```python
from build123d import *

# Parameters (mm, degrees)
BOSS_EXTRUDE1_DEPTH                             = 4.7625
CUT_EXTRUDE1_DEPTH                              = 98.916706472
FILLET1_R                                       = 3
M2_5X0_45_TAPPED_HOLE1_D                        = 2.05
M4X0_7_TAPPED_HOLE1_D                           = 3.3
M4X0_7_TAPPED_HOLE1_DEPTH                       = 11.5
M4X0_7_TAPPED_HOLE1_TIP                         = 0.991420021
CSK_FOR_M3_FLAT_HEAD_MACHINE_SCREW1_D           = 3.4
CSK_FOR_M3_FLAT_HEAD_MACHINE_SCREW1_CSINK_D     = 6.3
CSK_FOR_M3_FLAT_HEAD_MACHINE_SCREW1_CSINK_ANGLE = 90
CUT_EXTRUDE2_DEPTH                              = 84.778552935
FILLET2_R                                       = 2


with BuildPart() as part:
    # Sketch1 → Boss-Extrude1 (new, symmetric)
    with BuildSketch(Plane.XY):
        Polygon((-29.5, 68), (0, 78), (29.5, 68), (29.5, 0), (-29.5, 0), align=None)
    extrude(amount=BOSS_EXTRUDE1_DEPTH, both=True)

    # Sketch2 → Cut-Extrude1 (cut, through all)
    with BuildSketch(Plane(origin=(29.5, 0, 0), x_dir=(0, 0, -1), z_dir=(1, 0, 0))):
        Polygon((1.5875, 78), (1.5875, 15.875), (4.7625, 12.7), (4.7625, 78), align=None)
    extrude(amount=-CUT_EXTRUDE1_DEPTH, mode=Mode.SUBTRACT)

    # Fillet1
    fillet1_edges = [part.edges().sort_by_distance(p)[0] for p in [
        (0, 78, 1.5875),
        (29.5, 68, 1.5875),
        (29.5, 0, 0),
        (-29.5, 0, 0),
        (-29.5, 68, 1.5875),
    ]]
    fillet(fillet1_edges, radius=FILLET1_R)

    # M2.5x0.45 Tapped Hole1 (through all)
    with Locations(Plane.XY.offset(4.7625)):
        with Locations((-24.5, 5), (24.5, 5), (-24.5, 63), (24.5, 63)):
            Hole(M2_5X0_45_TAPPED_HOLE1_D / 2)

    # M4x0.7 Tapped Hole1
    with Locations(Plane(origin=(0, 0, 0), x_dir=(-1, 0, 0), z_dir=(0, -1, 0))):
        with Locations((-15, 0), (15, 0)):
            Hole(M4X0_7_TAPPED_HOLE1_D / 2, depth=M4X0_7_TAPPED_HOLE1_DEPTH)
            with Locations((0, 0, -(M4X0_7_TAPPED_HOLE1_DEPTH + M4X0_7_TAPPED_HOLE1_TIP / 2))):  # 118° drill point
                Cone(0, M4X0_7_TAPPED_HOLE1_D / 2, M4X0_7_TAPPED_HOLE1_TIP, mode=Mode.SUBTRACT)

    # CSK for M3 Flat Head Machine Screw1 (through all)
    with Locations(Plane.XY.offset(4.7625)):
        with Locations((-25.5, 28), (25.5, 28), (-25.5, 48), (25.5, 48)):
            CounterSinkHole(CSK_FOR_M3_FLAT_HEAD_MACHINE_SCREW1_D / 2, CSK_FOR_M3_FLAT_HEAD_MACHINE_SCREW1_CSINK_D / 2, counter_sink_angle=CSK_FOR_M3_FLAT_HEAD_MACHINE_SCREW1_CSINK_ANGLE)

    # Sketch7 → Cut-Extrude2 (cut, through all)
    with BuildSketch(Plane.XY.offset(4.7625)):
        with BuildLine():
            Line((-24.5, 43.101020514), (-24.5, 32.898979486))
            ThreePointArc((-24.5, 32.898979486), (-22.577443045, 32.056927513), (-21.169872981, 30.5))
            Line((-21.169872981, 30.5), (21.169872981, 30.5))
            ThreePointArc((21.169872981, 30.5), (22.577443045, 32.056927513), (24.5, 32.898979486))
            Line((24.5, 32.898979486), (24.5, 43.101020514))
            ThreePointArc((24.5, 43.101020514), (22.577443045, 43.943072487), (21.169872981, 45.5))
            Line((21.169872981, 45.5), (-21.169872981, 45.5))
            ThreePointArc((-21.169872981, 45.5), (-22.577443045, 43.943072487), (-24.5, 43.101020514))
        make_face()
        with BuildLine():
            ThreePointArc((-21.169872981, 25.5), (-22.577443045, 23.943072487), (-24.5, 23.101020514))
            Line((-24.5, 23.101020514), (-24.5, 10))
            ThreePointArc((-24.5, 10), (-22.263932023, 9.472135955), (-20.5, 8))
            Line((-20.5, 8), (-8, 8))
            Line((-8, 8), (-5, 5))
            Line((-5, 5), (5, 5))
            Line((5, 5), (8, 8))
            Line((8, 8), (20.5, 8))
            ThreePointArc((20.5, 8), (22.263932023, 9.472135955), (24.5, 10))
            Line((24.5, 10), (24.5, 23.101020514))
            ThreePointArc((24.5, 23.101020514), (22.577443045, 23.943072487), (21.169872981, 25.5))
            Line((21.169872981, 25.5), (-21.169872981, 25.5))
        make_face()
        with BuildLine():
            Line((-24.5, 58), (-24.5, 52.898979486))
            ThreePointArc((-24.5, 52.898979486), (-22.577443045, 52.056927513), (-21.169872981, 50.5))
            Line((-21.169872981, 50.5), (21.169872981, 50.5))
            ThreePointArc((21.169872981, 50.5), (22.577443045, 52.056927513), (24.5, 52.898979486))
            Line((24.5, 52.898979486), (24.5, 58))
            ThreePointArc((24.5, 58), (19.853737933, 61.15277267), (21.066919092, 66.635100477))
            Line((21.066919092, 66.635100477), (0, 73.776428982))
            Line((0, 73.776428982), (-21.066919092, 66.635100477))
            ThreePointArc((-21.066919092, 66.635100477), (-19.853737933, 61.15277267), (-24.5, 58))
        make_face()
    extrude(amount=-CUT_EXTRUDE2_DEPTH, mode=Mode.SUBTRACT)

    # Fillet2
    fillet2_edges = [part.edges().sort_by_distance(p)[0] for p in [
        (27, 15.875, -1.5875),
        (21.169872981, 50.5, 1.5875),
        (-21.169872981, 50.5, 1.5875),
        (-24.5, 52.898979486, 1.5875),
        (-24.5, 58, 1.5875),
        (-21.066919092, 66.635100477, 1.5875),
        (0, 73.776428982, 1.5875),
        (21.066919092, 66.635100477, 1.5875),
        (24.5, 58, 1.5875),
        (24.5, 52.898979486, 1.5875),
        (24.5, 43.101020514, 1.5875),
        (24.5, 32.898979486, 1.5875),
        (21.169872981, 30.5, 1.5875),
        (-21.169872981, 30.5, 1.5875),
        (-24.5, 32.898979486, 1.5875),
        (-24.5, 43.101020514, 1.5875),
        (-21.169872981, 45.5, 1.5875),
        (21.169872981, 45.5, 1.5875),
        (-24.5, 23.101020514, 1.5875),
        (-21.169872981, 25.5, 1.5875),
        (21.169872981, 25.5, 1.5875),
        (24.5, 23.101020514, 1.5875),
        (-24.5, 10, 0),
        (-8, 8, 0),
        (20.5, 8, 0),
        (24.5, 10, 0),
        (8, 8, 0),
        (5, 5, 0),
        (-5, 5, 0),
        (-20.5, 8, 0),
        (-27, 15.875, -1.5875),
    ]]
    fillet(fillet2_edges, radius=FILLET2_R)


solid = part.part
```
Verification items for the finished model (mm, model axes). Give positions to 0.01 mm unless a question says otherwise; leave off trailing zeros. Order: outer loops, then holes, each group sorted by start corner. A loop starts at its lowest first (then second) coordinate and runs counter-clockwise, first axis right, second up. Notation, with made-up numbers: M 50.25,-4 L 59.25,-4 A21 cw 59.25,8 Z; hole C -11,16 d5. An arc over 180 degrees is marked long. Return JSON: item names as keys, results as strings. Group by question number.
1) Section check A-A on y = 63. Record the cut outline in (x, z) (1 decimal), and give its area (3 significant figures).
2) Mould release check, pull along Y, two halves, no side actions. Record for faces 1 (the face through (0, 48, -1.588)), 2 (the face through (0, 0, 0)), 3 (the face through (-24, 53, 2)): pulls with the +Y half, pulls with the -Y half, needs draft (parallel to the pull), parting line crosses it, or undercut.
3) Section check B-B on y = 28. Record the cut outline in (x, z), and give its area (3 significant figures).
4) Scan lines: line 1 (X direction, y = 28, z = -0.45); line 2 (Y direction, x = 25, z = 1.75); line 3 (Y direction, x = 10.5, z = 4.25). Record each from-to range of solid material in increasing order.
5) Section check D-D on z = 0. Give the number of separate pieces and of enclosed holes in the cut face, and give its area (3 significant figures).
6) Go/stop test with flat-tipped pins: pin 1 Ø3 at (x, z) = (21, -1) entering from +Y; pin 2 Ø2 at (x, z) = (15, 0) entering from +Y; pin 3 Ø3 at (x, z) = (16, -2) entering from +Y; pin 4 Ø2 at (x, y) = (-25.5, 28) entering from +Z. Record where each tip stops, or that it passes through.
7) Section check C-C on x = 6.5. Record the cut outline in (y, z).
Answer block:
{
 "1": {"outline": "M -29.5,-1.6 L -25.5,-1.6 L -25.5,4.8 L -29.5,4.8 Z; M -23.5,-1.6 L -19.5,-1.6 L -19.5,4.8 L -23.5,4.8 Z; M 19.5,-1.6 L 23.5,-1.6 L 23.5,4.8 L 19.5,4.8 Z; M 25.5,-1.6 L 29.5,-1.6 L 29.5,4.8 L 25.5,4.8 Z", "area": "101 mm^2"},
 "2": {"face 1": "needs draft", "face 2": "pulls with the -Y half", "face 3": "undercut"},
 "3": {"outline": "M -29.5,-1.59 L -27.2,-1.59 L -27.2,3.31 L -28.65,4.76 L -29.5,4.76 Z; M -23.8,-1.59 L 23.8,-1.59 L 23.8,3.31 L 22.35,4.76 L -22.35,4.76 L -23.8,3.31 Z; M 27.2,-1.59 L 29.5,-1.59 L 29.5,4.76 L 28.65,4.76 L 27.2,3.31 Z", "area": "327 mm^2"},
 "4": {"line 1": "x = -29.5 to -27.2, -23.8 to 23.8, 27.2 to 29.5", "line 2": "y = 0 to 4.11, 5.89 to 26.38, 29.62 to 46.38, 49.62 to 62.11, 63.89 to 69.53", "line 3": "y = 0 to 8, 25.5 to 30.5, 45.5 to 50.5, 70.22 to 74.44"},
 "5": {"separate pieces": "2", "enclosed holes": "10", "area": "1,760 mm^2"},
 "6": {"pin 1": "stops at y = 71.39", "pin 2": "stops at y = 73.25", "pin 3": "stops at y = 73.07", "pin 4": "passes through"},
 "7": {"outline": "M 0,-4.76 L 6.5,-4.76 L 6.5,4.76 L 0,4.76 Z; M 25.5,-1.59 L 30.5,-1.59 L 30.5,4.76 L 25.5,4.76 Z; M 45.5,-1.59 L 50.5,-1.59 L 50.5,4.76 L 45.5,4.76 Z; M 71.57,-1.59 L 75.8,-1.59 L 75.8,4.76 L 71.57,4.76 Z"}
}
